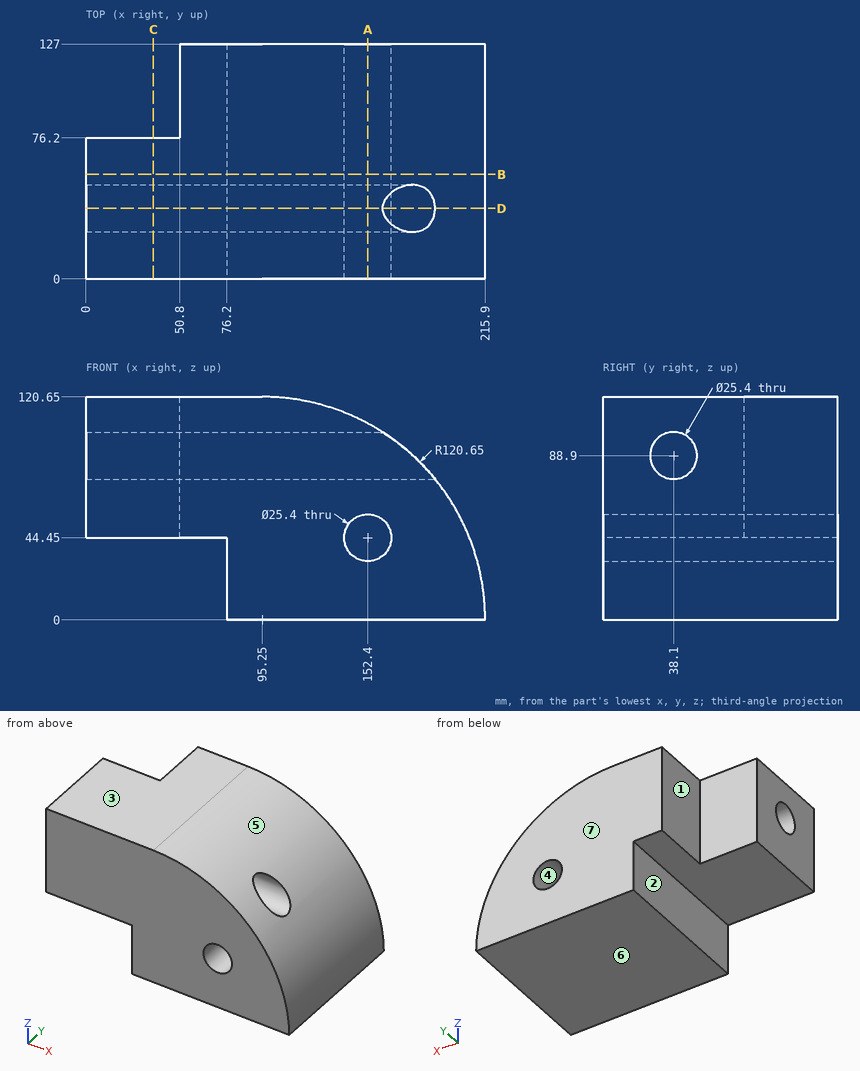
Study the drawing (mm; zero at the part's minimum x, y, z) and answer. A direction names the side the tool comes from. Coordinates: 2 decimals unless noted, no trailing zeros. Order: outer loops, then holes, each group sorted by start corner. A loop starts at its lowest first (then second) coordinate and runs counter-clockwise, first axis right, second up. Notation, with made-up numbers: (29.5, 63.5) -> (48.5, 63.5) arc R14 ccw to (48.5, 87.5) -> close; hole circle Ø8 at (31, 45). An arc over 180 degrees is marked (long way). Answer in a Markdown table with one row per item. Add a question column.
Item 1: Find section A-A (x = 152.4). Write down the section's boundary in (y, z).
Item 2: Find section D-D (y = 38.1). Write down the section's boundary in (x, z).
Item 3: Find section B-B (y = 56.5). Write down the section's boundary in (x, z), then the cut area to 3 significant figures.
Item 4: Which of the six approach directions +Z, -Z, +X, -X, +Y, -Y give full straight-line access (tool end or side, diameter ignored) to the marked faces 1, 2 and 3?
Item 5: Find the intervals of material crossed by L1, parallel to Z at x = 145, y = 38.1; L2, parallel to Z at x = 88, y = 38; L3, parallel to Z at x = 152.4, y = 42, in increasing order. Write a range as from..to.
Item 6: Determine the mould class of the marked faces 4, 5, 6 and 7 for opening direction Z: +Z half, -Z half, draft (parallel to the pull), parting line (faces both ways), or undercut.
Item 7: Each of these flat-tipped pins is pushed along its axis until it touches: P1, Ø23, axis at x = 34, y = 68.5, coming from the -Z side; P2, Ø15, axis at y = 102, z = 89.5, coming from the -X side; P3, Ø6, axis at y = 22, z = 107.5, coming from the +X side. Where does it stop, or does it pass through?
Item 8: Find section C-C (x = 36.5). Write down the section's boundary in (y, z), then the cut area to 3 significant figures.
Result set:
| question | item | result |
|---|---|---|
| 1 | outline | (0, 0) -> (127, 0) -> (127, 31.75) -> (0, 31.75) -> close; (0, 57.15) -> (127, 57.15) -> (127, 106.26) -> (0, 106.26) -> close; hole circle Ø25.4 at (38.1, 88.9) |
| 2 | outline | (0, 44.45) -> (76.2, 44.45) -> (76.2, 0) -> (215.9, 0) arc R120.65 ccw to (188.79, 76.2) -> (0, 76.2) -> close; (0, 101.6) -> (160.32, 101.6) arc R120.65 ccw to (95.25, 120.65) -> (0, 120.65) -> close; hole circle Ø25.4 at (152.4, 44.45) |
| 3 | outline | (0, 44.45) -> (76.2, 44.45) -> (76.2, 0) -> (215.9, 0) arc R120.65 ccw to (95.25, 120.65) -> (0, 120.65) -> close; hole circle Ø25.4 at (152.4, 44.45) |
| 3 | area | 19,000 mm² |
| 4 | face 1 | +Z, -Z, -X, +Y |
| 4 | face 2 | -Z, -X, +Y, -Y |
| 4 | face 3 | +Z, +X, -X, +Y, -Y |
| 5 | L1 | z = 0..34.13, 54.77..76.2, 101.6..109.92 |
| 5 | L2 | z = 0..76.2, 101.6..120.65 |
| 5 | L3 | z = 0..31.75, 57.15..76.81, 100.99..106.26 |
| 6 | face 4 | undercut |
| 6 | face 5 | +Z half |
| 6 | face 6 | -Z half |
| 6 | face 7 | draft |
| 7 | P1 | stops at z = 44.45 |
| 7 | P2 | stops at x = 50.8 |
| 7 | P3 | stops at x = 155.55 |
| 8 | outline | (0, 44.45) -> (76.2, 44.45) -> (76.2, 120.65) -> (0, 120.65) -> close; hole circle Ø25.4 at (38.1, 88.9) |
| 8 | area | 5,300 mm² |
